Work out the finished part from the listing and answer in its coordinate system (mm). A direction names the side the tool comes from. Coordinates: 2 decimals unless noted, no trailing zeros.
1. Determine the mould class of faces 1 (the flat face through (119, 19.05, 26)), 2 (the flat face through (119, 184.15, 48)), 3 (the flat face through (241.3, 94, 25)), 4 (the flat face through (119, 190.5, 26)) for opening direction X: +X half, -X half, draft (parallel to the pull), parting line (faces both ways), or undercut.
2. A tool of negligible diameter and unlimited length cuts with its end or side. For faces 5 (the flat face through (119, 0, 26)), 6 (the flat face through (6.35, 96, 3)), 7 (the flat face through (6.35, 94, 48)), 8 (the flat face through (19.05, 94, 26)), from which of +Z, -Z, +X, -X, +Y, -Y can it reach the whole face along a straight path? Write none if from no direction.
3. Find the intervals of material crossed by probe 1 along X at (y, z) = (150, 6.5); probe 2 along Y at (x, z) = (170.5, 20); probe 3 along X at (y, z) = (174, 2), in increasing order.
```python
from build123d import *

# Parameters (mm, degrees)
F0_W     = 241.3
F0_H     = 50.8
F1_DEPTH = 190.5
F2_W     = 203.2
F2_H     = 152.4
F3_DEPTH = 50.8
F4_W     = 228.6
F4_H     = 177.8
F5_DEPTH = 6.35
F6_W     = 228.6
F6_H     = 177.8
F7_DEPTH = 6.35
F8_R     = 1.5875


with BuildPart() as f1:
    # F0 (on Front) → F1 (new body)
    with BuildSketch(Plane.XZ):
        with Locations((120.65, 25.4)):
            Rectangle(F0_W, F0_H)
    extrude(amount=-F1_DEPTH)

    # F2 (on face) → F3 (cut, through all)
    with BuildSketch(Plane.XY.offset(50.8)):
        with Locations((120.65, 95.25)):
            Rectangle(F2_W, F2_H)
    extrude(amount=-F3_DEPTH, mode=Mode.SUBTRACT)

    # F4 (on face) → F5 (cut)
    with BuildSketch(Plane.XY.offset(50.8)):
        with Locations((120.65, 95.25)):
            Rectangle(F4_W, F4_H)
    extrude(amount=-F5_DEPTH, mode=Mode.SUBTRACT)

    # F6 (on face) → F7 (cut)
    with BuildSketch(Plane(origin=(0, 0, 0), x_dir=(1, 0, 0), z_dir=(0, 0, -1))):
        with Locations((120.65, -95.25)):
            Rectangle(F6_W, F6_H)
    extrude(amount=-F7_DEPTH, mode=Mode.SUBTRACT)

    # F8
    f8_edges = [f1.edges().sort_by_distance(p)[0] for p in [
        (120.65, 0, 50.8),
        (0, 0, 25.4),
        (0, 95.25, 50.8),
        (241.3, 0, 25.4),
        (241.3, 95.25, 50.8),
        (120.65, 190.5, 50.8),
        (241.3, 190.5, 25.4),
        (0, 190.5, 25.4),
        (120.65, 190.5, 0),
        (0, 95.25, 0),
        (120.65, 0, 0),
        (241.3, 95.25, 0),
    ]]
    fillet(f8_edges, radius=F8_R)


solid = f1.part
```
Geometry says:
1. face 1: undercut
1. face 2: undercut
1. face 3: +X half
1. face 4: draft
2. face 5: +Z, -Z, +X, -X, -Y
2. face 6: -Z
2. face 7: +Z
2. face 8: +Z, -Z
3. probe 1: x = 0 to 19.05, 222.25 to 241.3
3. probe 2: y = 0 to 19.05, 171.45 to 190.5
3. probe 3: x = 0 to 6.35, 234.95 to 241.3
